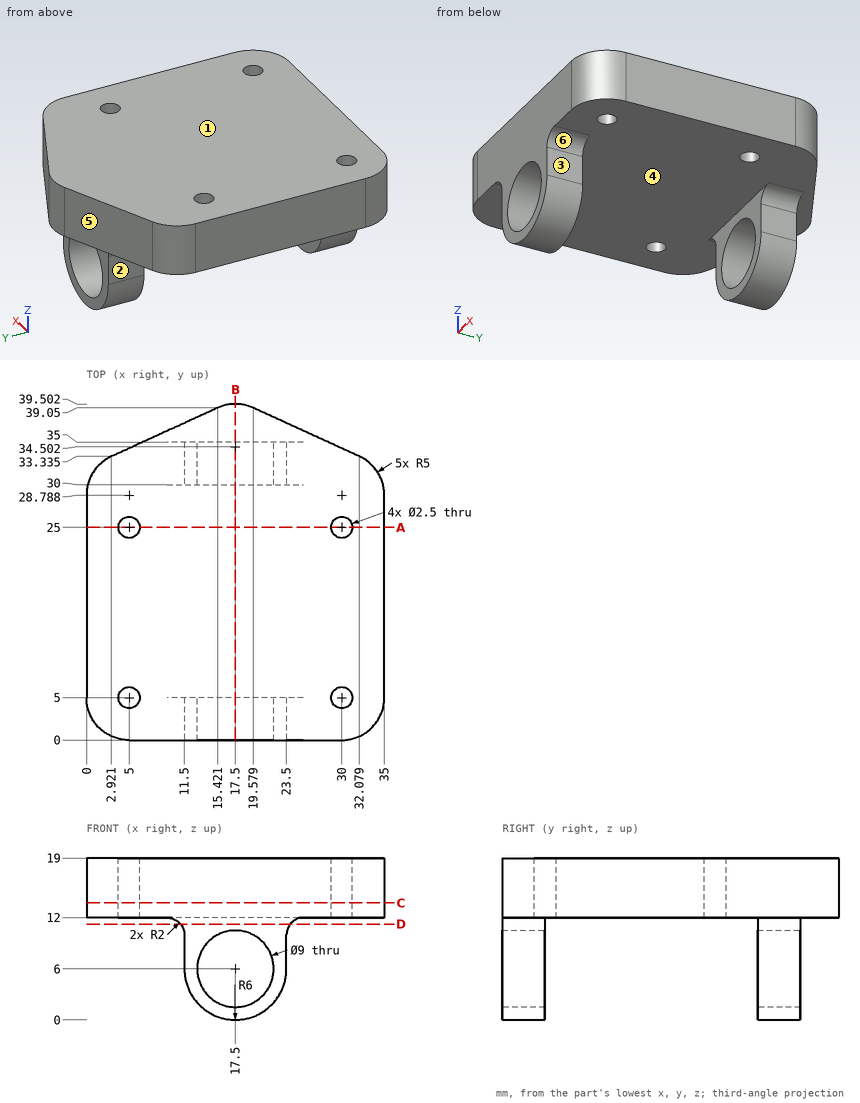
Job drawing, mm, ordinate dimensions from the low corner. One solid piece. A direction names the side the tool comes from. Round coordinates to 2 decimals unless told otherwise and drop trailing zeros. Loops run counter-clockwise (first coordinate to the right, second up) from the corner with the lowest first, then second, coordinate; pieces in that order, holes last.
(1) Cut at B-B (x = 17.5). Give the cut face in (y, z).
(2) Cut at C-C (z = 13.75). State how many separate pieces and enclosed holes the cut face has, plus the area to 3 significant figures.
(3) Cut at D-D (z = 11.25). Give the cut face in (x, y), plus the area to 3 significant figures.
(4) Cut at A-A (y = 25). Give the cut face in (x, z), plus the area to 3 significant figures.
(5) Drop flat-ended pins along their axis: pin 1 (3 mm diameter, centred on x = 5, y = 5, fed in from -Z); pin 2 (8 mm diameter, centred on x = 10.5, z = 13, fed in from +Y); pin 3 (1.2 mm diameter, centred on y = 31.5, z = 7, fed in from +X). Give the stop position or say it passes through.
(6) Two-plate mould, pull along Y, no slides. Class the marked faces 4, 5 and 6: +Y half, -Y half, draft (parallel to the pull), parting line (faces both ways), or undercut.
(7) Wall check: line 1 along X through (y, z) = (25, 16.75); line 2 along Y through (x, z) = (12.5, 5.5); line 3 along Y through (x, z) = (31, 12.25). Give the ranges that are in metal, low to high.
(8) Which spindle directions (+Z, -Z, +X, -X, +Y, -Y) get a long thin tool onto all of the face, cutting with end or side? Do the marked faces 1, 2 and 3. Say none if no direction does.
Findings below:
1. outline: (0, 0) - (5, 0) - (5, 1.5) - (0, 1.5) - close; (0, 10.5) - (5, 10.5) - (5, 12) - (30, 12) - (30, 10.5) - (35, 10.5) - (35, 12) - (39.5, 12) - (39.5, 19) - (0, 19) - close; (30, 0) - (35, 0) - (35, 1.5) - (30, 1.5) - close
2. separate pieces: 1
2. enclosed holes: 4
2. area: 1,230 mm2
3. outline: (11.06, 0) - (23.94, 0) - (23.94, 5) - (11.06, 5) - close; (11.06, 30) - (23.94, 30) - (23.94, 35) - (11.06, 35) - close
3. area: 129 mm2
4. outline: (0, 12) - (3.75, 12) - (3.75, 19) - (0, 19) - close; (6.25, 12) - (28.75, 12) - (28.75, 19) - (6.25, 19) - close; (31.25, 12) - (35, 12) - (35, 19) - (31.25, 19) - close
4. area: 210 mm2
5. pin 1: stops at z = 12
5. pin 2: stops at y = 38.63
5. pin 3: stops at x = 23.5
6. face 4: undercut
6. face 5: +Y half
6. face 6: draft
7. line 1: x = 0 to 3.75, 6.25 to 28.75, 31.25 to 35
7. line 2: y = 0 to 5, 30 to 35
7. line 3: y = 0.1 to 4.25, 5.75 to 24.25, 25.75 to 33.83
8. face 1: +Z, +X, -X, +Y, -Y
8. face 2: -Z, -X, +Y, -Y
8. face 3: -Z, +X, +Y, -Y
